Design review of the part built by this model. Coordinates are the model's own, in mm. Face numbers are marked on the shaded views. A direction names the side the tool comes from. Coordinates: 2 decimals unless noted, no trailing zeros. Order: outer loops, then holes, each group sorted by start corner. A loop starts at its lowest first (then second) coordinate and runs counter-clockwise, first axis right, second up. Notation, with made-up numbers: (22.25, 14.5) -> (37.25, 14.5) arc R33 ccw to (37.25, 44.5) -> close; hole circle Ø2 at (-17, -26). An arc over 180 degrees is marked (long way). Use a Markdown table: item, result. Add a question column.
Q1. Insertion check: pin 1 (4 mm diameter, centred on y = -0.5, z = 7, fed in from -X); pin 2 (1.5 mm diameter, centred on x = 21.5, y = -11.5, fed in from -Z). Each pin has a flat end and moves straight along its axis. Give the tip position at first contact, or say it passes through.
Q2. Add section B-B (z = 4.5). State the section outline as (x, y) points, then the cut area to 3 significant figures.
Q3. The part is to be moulded in two halves that separate along Y. For the marked faces 1, 2, 3 and 4, say which applies: pulls with the +Y half, pulls with the -Y half, needs draft (parallel to the pull), parting line crosses it, or undercut.
Q4. Add section A-A (y = -12). State the section outline as (x, z) points, then the cut area to 3 significant figures.
Q5. Add section C-C (y = 0). State the section outline as (x, z) points.
Q6. Machinability: for the marked faces 5, 6 and 7, which of the approach directions +Z, -Z, +X, -X, +Y, -Y give a long, thin tool a straight path to every point of the face, cutting with its end or side? Answer none if there is none.
Q7. Wall thickness on probe 1 along Y at (x, z) = (18, 1.25); probe 2 along Y at (x, z) = (28, 2.75); probe 3 along X at (y, z) = (15, 1.75): over which ranges is each line inside the solid? List them lowest first.
from build123d import *

# Parameters (mm, degrees)
CROQUIS1_R              = 3.5
SALIENTE_EXTRUIR2_DEPTH = 10


with BuildPart() as part:
    # Croquis1 → Saliente-Extruir2 (new body)
    with BuildSketch(Plane.XY):
        with BuildLine():
            Line((-30, 20), (30, 20))
            ThreePointArc((30, 20), (33.535533906, 18.535533906), (35, 15))
            Line((35, 15), (35, 5))
            Line((35, 5), (25, 5))
            ThreePointArc((25, 5), (20, 0), (25, -5))
            Line((25, -5), (35, -5))
            Line((35, -5), (35, -15))
            ThreePointArc((35, -15), (33.535533906, -18.535533906), (30, -20))
            Line((30, -20), (-30, -20))
            ThreePointArc((-30, -20), (-33.535533906, -18.535533906), (-35, -15))
            Line((-35, -15), (-35, -5))
            Line((-35, -5), (-25, -5))
            ThreePointArc((-25, -5), (-20, 0), (-25, 5))
            Line((-25, 5), (-35, 5))
            Line((-35, 5), (-35, 15))
            ThreePointArc((-35, 15), (-33.535533906, 18.535533906), (-30, 20))
        make_face()
        with Locations((20, 12)):
            Circle(CROQUIS1_R, mode=Mode.SUBTRACT)
        with Locations(Location((20, -12, 0), (0, 0, 180))):
            Circle(CROQUIS1_R, mode=Mode.SUBTRACT)
        with Locations((-20, -12)):
            Circle(CROQUIS1_R, mode=Mode.SUBTRACT)
        with Locations(Location((-20, 12, 0), (0, 0, 180))):
            Circle(CROQUIS1_R, mode=Mode.SUBTRACT)
    extrude(amount=SALIENTE_EXTRUIR2_DEPTH)


solid = part.part
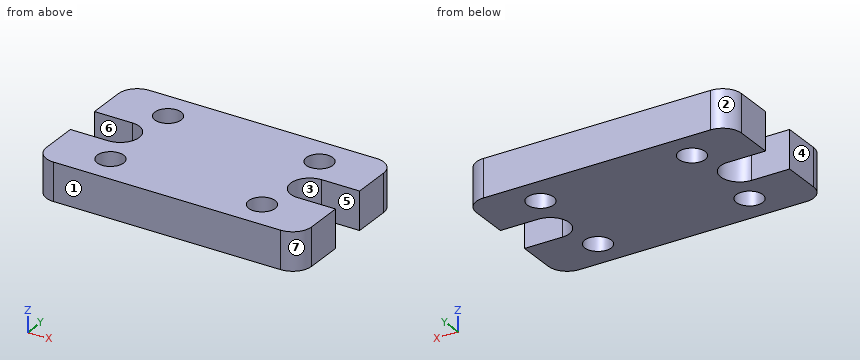
Established:
| question | item | result |
|---|---|---|
| 1 | pin 1 | x = -20.67 |
| 1 | pin 2 | through |
| 2 | outline | (-35, -15) arc R5 ccw to (-30, -20) -> (30, -20) arc R5 ccw to (35, -15) -> (35, -5) -> (25, -5) arc R5 cw to (25, 5) -> (35, 5) -> (35, 15) arc R5 ccw to (30, 20) -> (-30, 20) arc R5 ccw to (-35, 15) -> (-35, 5) -> (-25, 5) arc R5 cw to (-25, -5) -> (-35, -5) -> close; hole circle Ø7 at (-20, -12); hole circle Ø7 at (-20, 12); hole circle Ø7 at (20, -12); hole circle Ø7 at (20, 12) |
| 2 | area | 2,350 mm^2 |
| 3 | face 1 | pulls with the -Y half |
| 3 | face 2 | pulls with the +Y half |
| 3 | face 3 | undercut |
| 3 | face 4 | needs draft |
| 4 | outline | (-35, 0) -> (-23.5, 0) -> (-23.5, 10) -> (-35, 10) -> close; (-16.5, 0) -> (16.5, 0) -> (16.5, 10) -> (-16.5, 10) -> close; (23.5, 0) -> (35, 0) -> (35, 10) -> (23.5, 10) -> close |
| 4 | area | 560 mm^2 |
| 5 | outline | (-20, 0) -> (20, 0) -> (20, 10) -> (-20, 10) -> close |
| 6 | face 5 | +Z, -Z, +X |
| 6 | face 6 | +Z, -Z, -X |
| 6 | face 7 | +Z, -Z, +X, -Y |
| 7 | probe 1 | -20 to -14.87, -9.13 to 9.13, 14.87 to 20 |
| 7 | probe 2 | -20 to -5, 5 to 20 |
| 7 | probe 3 | -35 to -21.8, -18.2 to 18.2, 21.8 to 35 |
